```python
from build123d import *

# Parameters (mm, degrees)
SKETCH_W        = 94
SKETCH_H        = 68.7
SKETCH_R        = 1.6
PAD_DEPTH       = 6
SKETCH001_W     = 22
SKETCH001_H     = 17
SKETCH001_W_2   = 17.9
SKETCH001_H_2   = 15.1
POCKET_DEPTH    = 6
POCKET001_DEPTH = 3
FILLET_R        = 4


with BuildPart() as part:
    # Sketch → Pad (new body)
    with BuildSketch(Plane.XY):
        with Locations((47, 34.35)):
            Rectangle(SKETCH_W, SKETCH_H)
        with Locations((3.45, 65.25)):
            Circle(SKETCH_R, mode=Mode.SUBTRACT)
        with Locations((90.55, 65.25)):
            Circle(SKETCH_R, mode=Mode.SUBTRACT)
        with Locations((90.55, 3.45)):
            Circle(SKETCH_R, mode=Mode.SUBTRACT)
        with Locations((3.45, 3.45)):
            Circle(SKETCH_R, mode=Mode.SUBTRACT)
    extrude(amount=PAD_DEPTH)

    # Sketch001 (on Face10 of Pad) → Pocket (cut)
    with BuildSketch(Plane.XY.offset(6)):
        with Locations((11, 16.7)):
            Rectangle(SKETCH001_W, SKETCH001_H)
        with Locations((8.95, 35.55)):
            Rectangle(SKETCH001_W_2, SKETCH001_H_2)
        with Locations((8.95, 53.45)):
            Rectangle(SKETCH001_W_2, SKETCH001_H_2)
        with BuildLine():
            Line((92, 43.6), (92, 25.1))
            ThreePointArc((94, 23.1), (93.414214, 24.514214), (92, 25.1))
            Line((94, 23.1), (94, 45.6))
            ThreePointArc((92, 43.6), (93.414214, 44.185786), (94, 45.6))
        make_face()
        with BuildLine():
            Line((88.5, 68.7), (88.5, 62.2))
            Line((88.5, 62.2), (82.3, 62.2))
            Line((82.3, 62.2), (82.3, 54.05))
            Line((82.3, 54.05), (88.5, 54.05))
            Line((88.5, 54.05), (88.5, 6.8))
            ThreePointArc((88, 6.3), (88.353553, 6.446447), (88.5, 6.8))
            Line((88, 6.3), (26.5, 6.3))
            ThreePointArc((26, 6.8), (26.146447, 6.446447), (26.5, 6.3))
            Line((26, 6.8), (26, 11.5))
            Line((26, 11.5), (23.5, 11.5))
            Line((23.5, 11.5), (23.5, 52.9))
            Line((23.5, 52.9), (29.5, 52.9))
            Line((29.5, 52.9), (29.5, 62.2))
            Line((29.5, 62.2), (23.5, 62.2))
            Line((23.5, 62.2), (23.5, 68.7))
            Line((23.5, 68.7), (88.5, 68.7))
        make_face()
    extrude(amount=-POCKET_DEPTH, mode=Mode.SUBTRACT)

    # Sketch002 (on Face4 of Pocket) → Pocket001 (cut)
    with BuildSketch(Plane(origin=(0, 0, 0), x_dir=(1, 0, 0), z_dir=(0, 0, -1))):
        Polygon((22, -18.1), (23.5, -18.1), (23.5, -31.2), (22.5, -31.2), (22.5, -33.2), (17.9, -33.2), (17.9, -28), (0, -28), (0, -25.2), (22, -25.2), align=None)
        Polygon((0, -43.1), (23.5, -43.1), (23.5, -58.2), (20.9, -58.2), (20.9, -61), (17.9, -61), (17.9, -45.9), (0, -45.9), align=None)
    extrude(amount=-POCKET001_DEPTH, mode=Mode.SUBTRACT)

    # Fillet
    fillet_edges = [part.edges().sort_by_distance(p)[0] for p in [
        (0, 68.7, 3),
        (0, 0, 3),
        (94, 0, 3),
        (94, 68.7, 3),
    ]]
    fillet(fillet_edges, radius=FILLET_R)


solid = part.part
```
The model under review builds one solid part; all positions refer to its coordinate system, in mm. A direction names the side the tool comes from. Round coordinates to 2 decimals unless told otherwise and drop trailing zeros. Write each loop counter-clockwise with the first axis right and the second up, starting at its lowest first coordinate (ties: lowest second). Pieces come first, ordered by that corner, then holes. Notation, with made-up numbers: (52.25, -28.5) -> (97.25, -28.5) arc R18 cw to (97.25, -18.5) -> close; hole circle Ø7 at (47, -17). An arc over 180 degrees is marked (long way). Use CSV: the item, a comma, the result in double quotes.
Q1. For pin 1 Ø1.8 at (y, z) = (59.5, 4) entering from -X; pin 2 Ø1.5 at (y, z) = (20, 2.5) entering from -X; pin 3 Ø12 at (x, y) = (16.5, 23.5) entering from -Z, all flat-tipped, find the tip position at first contact; note any pin that passes through.
Checks:
pin 1,"x = 17.9"
pin 2,"x = 22"
pin 3,"z = 3"
Q2. Consider section D-D (y = 55.5). Give the boundary of the cut face in (x, z).
Checks:
outline,"(17.9, 3) -> (23.5, 3) -> (23.5, 0) -> (29.5, 0) -> (29.5, 6) -> (17.9, 6) -> close; (82.3, 0) -> (94, 0) -> (94, 6) -> (82.3, 6) -> close"
Q3. To check wall thickness, follow probe 1 along Y at (x, z) = (13, 4.05); probe 2 along X at (y, z) = (54, 2.25); probe 3 along X at (y, z) = (52.5, 4.8). State the ranges of each line that lie inside material, in increasing order. Write a range as [from, to].
Checks:
probe 1,"[0, 8.2], [25.2, 28], [43.1, 45.9], [61, 68.7]"
probe 2,"[23.5, 29.5], [88.5, 94]"
probe 3,"[17.9, 23.5], [88.5, 94]"
Q4. Consider section A-A (y = 39). Give the boundary of the cut face in (x, z).
Checks:
outline,"(17.9, 0) -> (23.5, 0) -> (23.5, 6) -> (17.9, 6) -> close; (88.5, 0) -> (92, 0) -> (92, 6) -> (88.5, 6) -> close"
Q5. For faces 1 (the flat face through (9, 43.1, 5)), 2 (the flat face through (26, 9, 3)), 3 (the flat face through (82.3, 58, 3)), 4 (the flat face through (21, 43.1, 1)), list the 3-axis set-ups (+Z, -Z, +X, -X, +Y, -Y) from which the entire face can be reached by the end or side of a thin tool; tool diameter is ignored.
Checks:
face 1,"+Z, -Z, -X"
face 2,"+Z, -Z"
face 3,"+Z, -Z, +Y"
face 4,"-Z, -X"
Q6. Consider section C-C (x = 49.5). Give the boundary of the cut face in (y, z), then the cut area to 3 significant figures.
Checks:
outline,"(0, 0) -> (6.3, 0) -> (6.3, 6) -> (0, 6) -> close"
area,"37.8 mm²"
Q7. Consider section B-B (z = 1.65). State how many separate pieces and enclosed holes the cut face has, then the cut area to 3 significant figures.
Checks:
separate pieces,"3"
enclosed holes,"4"
area,"1,280 mm²"
